The listing builds one solid part. Answer for the finished solid, in the listing's coordinates (mm). Face numbers are marked on the shaded views. A direction names the side the tool comes from. Round coordinates to 2 decimals unless told otherwise and drop trailing zeros. Write each loop counter-clockwise with the first axis right and the second up, starting at its lowest first coordinate (ties: lowest second). Pieces come first, ordered by that corner, then holes. Notation, with made-up numbers: M -39.75,81.25 L -32.75,81.25 A9 ccw -32.75,89.25 Z; hole C -24.5,70 d9. An arc over 180 degrees is marked long. One line per item, written item: value. Start each with the question number.
(1) Section A-A (z = 31) is taken. Determine the outline of the cut face in (x, y) (3 decimals).
(2) Given P1, Ø3, axis at y = -1.5, z = 30.5, coming from the +X side; P2, Ø3, axis at x = 2, z = 25, coming from the -Y side; P3, Ø0.8, axis at y = 0.5, z = 31, coming from the +X side; P4, Ø2.5, axis at x = 0.5, y = 0, coming from the +Z side, each flat-ended and moving along its own axis, determine where each tip first touches the part or whether it passes through.
(3) For the marked faces 1 and 2, determine the directions among +Z, -Z, +X, -X, +Y, -Y from which every point of the face is accessible in a straight line to the end or side of a thin tool.
(4) For a pull along X with two mould halves and no side action, classify the marked faces 3, 4 and 5 as released by +X, released by -X, zero draft, split by the parting line, or undercut.
(5) Consider probe 1 along X at (y, z) = (0.25, 31) (3 decimals); probe 2 along Y at (x, z) = (0, 27.5); probe 3 along X at (y, z) = (-1.4, 31.25). Determine where each line is inside the solid, lowest interval first.
(6) Section C-C (z = 26) is taken. Determine the outline of the cut face in (x, y).
(7) Section B-B (y = 0) is taken. Determine the outline of the cut face in (x, z) (3 decimals).
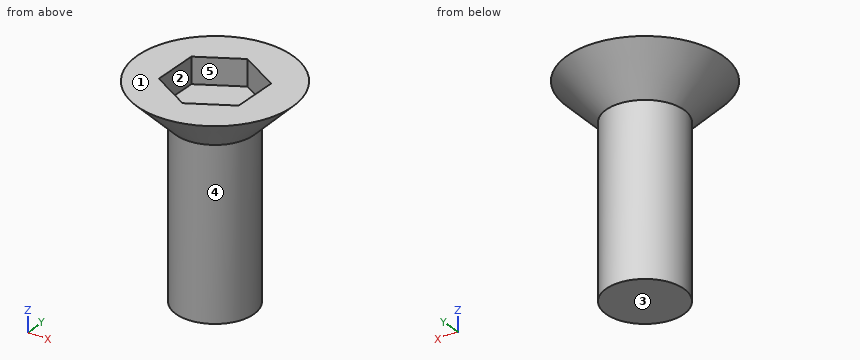
Solid Edge part; units mm, degrees
sketch "Sketch1" plane through (0, 0, 0) normal (0, 0, 1) x (1, 0, 0)
  circle A0 centre (0, 0) radius 1.5
extrude "Protrusion1" add sketch "Sketch1" along normal blind 30
sketch "Sketch2" plane through (0, 0, 30) normal (0, 0, 1) x (1, 0, 0)
  circle A0 centre (0, 0) radius 3
extrude "ExtrudedProtrusion_2" add sketch "Sketch2" along normal blind 1.75
chamfer "Chamfer_1" distance 1.75 angle 45 1 edges at (-3, 0, 30)
sketch "Sketch3" plane through (0, 0, 31.75) normal (0, 0, 1) x (0, 1, 0)
  line L0 (0.8978, -1.555) -> (1.7956, 0)
  line L1 (1.7956, 0) -> (0.8978, 1.555)
  line L2 (0.8978, 1.555) -> (-0.8978, 1.555)
  line L3 (-0.8978, 1.555) -> (-1.7956, 0)
  line L4 (-1.7956, 0) -> (-0.8978, -1.555)
  line L5 (-0.8978, -1.555) -> (0.8978, -1.555)
extrude "ExtrudedCutout_1" cut sketch "Sketch3" against normal blind 1
sketch "Sketch4" plane through (0, 0, 0) normal (0, 0, -1) x (0, 1, 0)
  circle A0 centre (0, 0) radius 1.9215
extrude "ExtrudedCutout_2" cut sketch "Sketch4" against normal blind 23.75
revolve "RevolvedCutout1" [suppressed]
fillet "Round_1" [suppressed]
properties material "Iron, grey cast type 20"
Recorded:
1. outline: C 0,0 d4.5; hole M -1.555,-0.898 L 0,-1.796 L 1.555,-0.898 L 1.555,0.898 L 0,1.796 L -1.555,0.898 Z
2. P1: stops at x = 2.92
2. P2: stops at y = -1.41
2. P3: stops at x = 2.61
2. P4: stops at z = 31.75
3. face 1: +Z, +X, -X, +Y, -Y
3. face 2: +Z
4. face 3: zero draft
4. face 4: split by the parting line
4. face 5: undercut
5. probe 1: x = -2.236 to -1.555, 1.555 to 2.236
5. probe 2: y = -1.5 to 1.5
5. probe 3: x = -2.07 to -0.69, 0.69 to 2.07
6. outline: C 0,0 d3
7. outline: M -3,31.75 L -1.5,30.25 L -1.5,23.75 L 1.5,23.75 L 1.5,30.25 L 3,31.75 L 1.555,31.75 L 1.555,30.75 L -1.555,30.75 L -1.555,31.75 Z
